```python
from build123d import *

# Parameters (mm, degrees)
SKETCH_1_R          = 5.5
SKETCH_1_R_2        = 1.5
EXTRUDE_2_DEPTH     = 5
CUT_EXTRUDE_1_DEPTH = 33.746182984


with BuildPart() as part:
    # Эскиз1 → Бобышка-Вытянуть2 (new body)
    with BuildSketch(Plane(origin=(0, 0, 0), x_dir=(1, 0, 0), z_dir=(0, 1, 0))):
        with BuildLine():
            ThreePointArc((-8.362025498, 1.525296552), (-0.667373394, -8.473760249), (8.497706046, 0.197463815))
            Line((8.497706046, 0.197463815), (16.18697839, 1.21124957))
            Line((16.18697839, 1.21124957), (30.25, 9))
            Line((30.25, 9), (30.25, 10.5))
            Line((30.25, 10.5), (29, 11.5))
            Line((29, 11.5), (27.75, 10.5))
            Line((27.75, 10.5), (26.5, 11.5))
            Line((26.5, 11.5), (25.25, 10.5))
            Line((25.25, 10.5), (24, 11.5))
            Line((24, 11.5), (22.75, 10.5))
            Line((22.75, 10.5), (21.5, 11.5))
            Line((21.5, 11.5), (20.25, 10.5))
            Line((20.25, 10.5), (19, 11.5))
            Line((19, 11.5), (18, 11.5))
            ThreePointArc((18, 11.5), (15, 8.5), (12, 11.5))
            Line((12, 11.5), (3.296389157, 7.834782609))
            ThreePointArc((3.296389157, 7.834782609), (2.077275401, 8.776959062), (1.486606875, 10.2))
            ThreePointArc((1.486606875, 10.2), (0.987420883, 11.129158979), (0, 11.5))
            ThreePointArc((0, 11.5), (-6.242051456, 9.658508871), (-10.485027716, 4.723790195))
            Line((-10.485027716, 4.723790195), (-8.731080367, 2.807108505))
            ThreePointArc((-8.731080367, 2.807108505), (-8.396232651, 2.209482225), (-8.362025498, 1.525296552))
        make_face()
        with Locations(Location((0, 0, 0), (0, 0, 270))):
            Circle(SKETCH_1_R, mode=Mode.SUBTRACT)
        with Locations(Location((-6.480740698, 5.5, 0), (0, 0, 270))):
            Circle(SKETCH_1_R_2, mode=Mode.SUBTRACT)
    extrude(amount=EXTRUDE_2_DEPTH)

    # Эскиз2 → Вырез-Вытянуть1 (cut, through all)
    with BuildSketch(Plane(origin=(0, 5, 0), x_dir=(1, 0, 0), z_dir=(0, 1, 0))):
        with BuildLine():
            ThreePointArc((-9.310541114, 3.440332646), (-9.842132841, 4.524785735), (-9.973477908, 5.72535924))
            ThreePointArc((-9.973477908, 5.72535924), (-10.241503709, 5.230831844), (-10.485027716, 4.723790195))
            Line((-10.485027716, 4.723790195), (-9.310541114, 3.440332646))
        make_face()
    extrude(amount=-CUT_EXTRUDE_1_DEPTH, mode=Mode.SUBTRACT)


solid = part.part
```
For this review, take the finished solid that the model builds, in its own axes (mm). A direction names the side the tool comes from. Round coordinates to 2 decimals unless told otherwise and drop trailing zeros. Loops run counter-clockwise (first coordinate to the right, second up) from the corner with the lowest first, then second, coordinate; pieces in that order, holes last.
Q1. Add section D-D on x = 21. Write out the cut boundary in (y, z), plus the area to 3 significant figures.
Result sheet:
outline: (0, -11.1) - (5, -11.1) - (5, -3.88) - (0, -3.88) - close
area: 36.1 mm2
Q2. Mouldability with a two-part tool opening along Z and no side actions: class faces 1 (the face through (23.12, 2.46, -5.05)), 2 (the face through (15.1, 2.5, -8.5)), 3 (the face through (5, 0, -4)), 4 (the face through (-5.47, 2.46, -6.61)) as +Z half, -Z half, draft (parallel to the pull), parting line (faces both ways), or undercut.
Result sheet:
face 1: +Z half
face 2: -Z half
face 3: draft
face 4: undercut
Q3. Add section B-B on x = 1. Write out the cut boundary in (y, z).
Result sheet:
outline: (0, -11.12) - (5, -11.12) - (5, -5.41) - (0, -5.41) - close; (0, 5.41) - (5, 5.41) - (5, 8.44) - (0, 8.44) - close
Q4. Add section C-C on y = 4.2. Write out the cut boundary in (x, z).
Result sheet:
outline: (-9.97, -5.73) arc R11.5 ccw to (0, -11.5) arc R1.5 ccw to (1.49, -10.2) arc R3 cw to (3.3, -7.83) - (12, -11.5) arc R3 cw to (18, -11.5) - (19, -11.5) - (20.25, -10.5) - (21.5, -11.5) - (22.75, -10.5) - (24, -11.5) - (25.25, -10.5) - (26.5, -11.5) - (27.75, -10.5) - (29, -11.5) - (30.25, -10.5) - (30.25, -9) - (16.19, -1.21) - (8.5, -0.2) arc R8.5 ccw (long way) to (-8.36, -1.53) arc R1.5 cw to (-8.73, -2.81) - (-9.31, -3.44) arc R3.5 ccw to start; hole circle Ø3 at (-6.48, -5.5); hole circle Ø11 at (0, 0)
Q5. Machinability: for faces 5 (the face through (19.634, 2.465, -10.993)), 6 (the face through (30.25, 2, -10)), which of the approach directions +Z, -Z, +X, -X, +Y, -Y give a long, thin tool a straight path to every point of the face, cutting with its end or side? Answer none if there is none.
Result sheet:
face 5: -Z, +Y, -Y
face 6: +Z, -Z, +X, +Y, -Y
Q6. To check wall thickness, follow line 1 along X through (y, z) = (3.05, -5); line 2 along X through (y, z) = (2.2, 0); line 3 along Z through (x, y) = (-3, 3.85). State the ranges of each line that lie inside material, in increasing order.
Result sheet:
line 1: x = -9.94 to -7.89, -5.07 to -2.29, 2.29 to 23.03
line 2: x = -8.5 to -5.5, 5.5 to 8.5
line 3: z = -11.1 to -4.61, 4.61 to 7.95
Q7. Add section A-A on z = -4.5. Write out the cut boundary in (x, y) (3 decimals), plus the area to 3 significant figures.
Result sheet:
outline: (-9.835, 0) - (-7.599, 0) - (-7.599, 5) - (-9.835, 5) - close; (-5.363, 0) - (-3.162, 0) - (-3.162, 5) - (-5.363, 5) - close; (3.162, 0) - (22.125, 0) - (22.125, 5) - (3.162, 5) - close
area: 117 mm2
